Work out the finished part from the listing and answer in its coordinate system (mm). Face numbers are marked on the shaded views. A direction names the side the tool comes from. Round coordinates to 2 decimals unless told otherwise and drop trailing zeros. Loops run counter-clockwise (first coordinate to the right, second up) from the corner with the lowest first, then second, coordinate; pieces in that order, holes last. Notation, with made-up numbers: (26, 30.5) -> (65, 30.5) arc R28 ccw to (65, 53.5) -> close; hole circle Ø11 at (68.5, 17). An arc over 180 degrees is marked (long way). Use CSV: the item, a comma, the result in double quotes. Start each with the question number.
Autodesk Inventor part; units mm, degrees
ref_plane "YZ Plane" through (0, 0, 0) normal (1, 0, 0) x (0, 1, 0)
ref_plane "XZ Plane" through (0, 0, 0) normal (0, 1, 0) x (-1, 0, 0)
ref_plane "XY Plane" through (0, 0, 0) normal (0, 0, 1) x (1, 0, 0)
sketch "スケッチ1" plane through (0, 0, 0) normal (1, 0, 0) x (0, 1, 0)
  line L0 (1.7321, -3) -> (-1.7321, -3)
  line L1 (-1.7321, -3) -> (-3.4641, 0)
  line L2 (-3.4641, 0) -> (-1.7321, 3)
  line L3 (-1.7321, 3) -> (1.7321, 3)
  line L4 (1.7321, 3) -> (3.4641, 0)
  line L5 (3.4641, 0) -> (1.7321, -3)
  point P0 (0, 0)
  point P1 (0, 0)
  dimension "d0" = 6
extrude "押し出し1" add sketch "スケッチ1" along normal blind 40
sketch "スケッチ2" plane through (40, 0, 0) normal (1, 0, 0) x (0, 0, -1)
  circle A0 centre (0, 0) radius 2
  dimension "d3" = 4
extrude "押し出し2" add sketch "スケッチ2" along normal blind 8
thread "ねじ1"
sketch "スケッチ3" plane through (0, 0, 0) normal (-1, 0, 0) x (0, 0, 1)
  point P0 (0, 0)
  point P1 (0, 0)
hole "穴1" at (0, 0, 0) direction (1, 0, 0) diameter 3.242 depth 11.8 tip angle 118
properties part number "Spacer_M3_L15" material "鋼、合金"
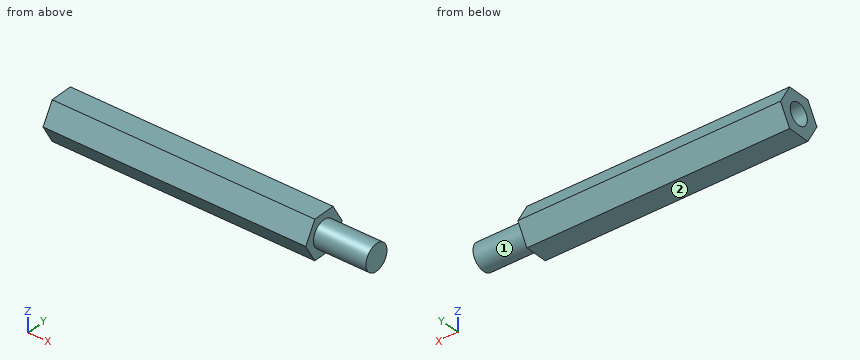
Q1. Each of these flat-tipped pins is pushed along its axis until it touches: pin 1 (1.5 mm diameter, centred on x = 6.5, z = 2, fed in from -Y); pin 2 (3 mm diameter, centred on y = 0, z = 0, fed in from -X); pin 3 (1 mm diameter, centred on y = -0.5, z = 0, fed in from -X). Where does it stop, or does it pass through?
Q2. Section A-A, the plane x = 16.5 is taken. Write down the section's boundary in (y, z).
Q3. Straight lines are drawn through the part: line 1 (Y direction, x = 4.5, z = 0); line 2 (Z direction, x = 8.5, y = 0); line 3 (X direction, y = 0, z = -2.2). For each, find the intervals that lie inside material, in ascending order. Write a range as from..to.
Q4. Which of the six approach directions +Z, -Z, +X, -X, +Y, -Y give full straight-line access (tool end or side, diameter ignored) to the marked faces 1 and 2?
Report:
1,pin 1,"stops at y = -2.74"
1,pin 2,"stops at x = 11.87"
1,pin 3,"stops at x = 12.17"
2,outline,"(-3.46, 0) -> (-1.73, -3) -> (1.73, -3) -> (3.46, 0) -> (1.73, 3) -> (-1.73, 3) -> close"
3,line 1,"y = -3.46..-1.62, 1.62..3.46"
3,line 2,"z = -3..-1.62, 1.62..3"
3,line 3,"x = 0..40"
4,face 1,"+X"
4,face 2,"-Z, +X, -X, +Y, -Y"
